Verification items for the finished model (mm, model axes). A direction names the side the tool comes from. Give positions to 0.01 mm unless a question says otherwise; leave off trailing zeros. Order: outer loops, then holes, each group sorted by start corner. A loop starts at its lowest first (then second) coordinate and runs counter-clockwise, first axis right, second up. Notation, with made-up numbers: (41.25, -13) -> (49.25, -13) arc R16 cw to (49.25, -6) -> close; hole circle Ø6 at (-32, -3.75). An arc over 180 degrees is marked (long way). Write each question's results on one line, items separated by ' | '. Start each with the question number.
1. Set-up check for faces 1 (the face through (2.5, 1, 3)), 2 (the face through (25.5, 1, 3)), 3 (the face through (22.024, 1.014, 2.283)): record each of +Z, -Z, +X, -X, +Y, -Y from which the full face is reachable in a straight line by a thin tool's end or side.
2. Cross-section at A-A, the plane x = 23. Enter the section's corners in (y, z), then the cut area to 3 significant figures.
3. Cross-section at D-D, the plane x = 5. Enter the section's corners in (y, z).
4. Material ranges on L1, parallel to X at y = 0.9, z = -3; L2, parallel to X at y = 0.85, z = -4; L3, parallel to Z at x = 5.5, y = 0.4, recorded low to high. Write a range as from..to.
5. Cross-section at B-B, the plane z = -3. Enter the section's corners in (x, y), then the cut area to 3 significant figures.
6. Depth check by flat-ended pin: pin 1 Ø0.6 at (y, z) = (1, 2) entering from -X; pin 2 Ø0.6 at (x, y) = (27, 1) entering from +Z. Enter the tip coordinate at first touch or a pass-through.
7. Cross-section at C-C, the plane y = 1.3. Enter the section's corners in (x, z), then the cut area to 3 significant figures.
8. Mould release check, pull along Z, two halves, no side actions. Record for faces 4 (the face through (0, 1, -3)), 5 (the face through (5.676, 1.014, 1.763)), 6 (the face through (15, 1, -6)), 7 (the face through (14, 1, 5)): +Z half, -Z half, draft (parallel to the pull), parting line (faces both ways), or undercut.
from build123d import *

# Parameters (mm, degrees)
SKETCH_1_W      = 30
SKETCH_1_H      = 6
SKETCH_1_R      = 1.5
EXTRUDE_1_DEPTH = 2
SKETCH_2_W      = 23
SKETCH_2_H      = 5
SKETCH_2_R      = 1
EXTRUDE_2_DEPTH = 2


with BuildPart() as part:
    # 草图1 → 凸台-拉伸1 (new body)
    with BuildSketch(Plane(origin=(0, 0, 0), x_dir=(1, 0, 0), z_dir=(0, 1, 0))):
        with Locations((15, 3)):
            Rectangle(SKETCH_1_W, SKETCH_1_H)
        with Locations(Location((5, 3, 0), (0, 0, 270))):
            Circle(SKETCH_1_R, mode=Mode.SUBTRACT)
        with Locations(Location((25, 3, 0), (0, 0, 270))):
            Circle(SKETCH_1_R, mode=Mode.SUBTRACT)
    extrude(amount=EXTRUDE_1_DEPTH)

    # 草图2 → 凸台-拉伸2 (add)
    with BuildSketch(Plane(origin=(0, 2, 0), x_dir=(1, 0, 0), z_dir=(0, 1, 0))):
        with Locations((14, -2.5)):
            Rectangle(SKETCH_2_W, SKETCH_2_H)
        with Locations(Location((5, -2.5, 0), (0, 0, 270))):
            Circle(SKETCH_2_R, mode=Mode.SUBTRACT)
        with Locations(Location((23, -2.5, 0), (0, 0, 270))):
            Circle(SKETCH_2_R, mode=Mode.SUBTRACT)
    extrude(amount=-EXTRUDE_2_DEPTH)


solid = part.part
Results below:
1) face 1: +Z, -X, +Y, -Y | face 2: +Z, +X, +Y, -Y | face 3: +Y, -Y
2) outline: (0, -6) -> (2, -6) -> (2, 1.5) -> (0, 1.5) -> close; (0, 3.5) -> (2, 3.5) -> (2, 5) -> (0, 5) -> close | area: 18.0 mm²
3) outline: (0, -6) -> (2, -6) -> (2, -4.5) -> (0, -4.5) -> close; (0, -1.5) -> (2, -1.5) -> (2, 1.5) -> (0, 1.5) -> close; (0, 3.5) -> (2, 3.5) -> (2, 5) -> (0, 5) -> close
4) L1: x = 0..3.5, 6.5..23.5, 26.5..30 | L2: x = 0..3.88, 6.12..23.88, 26.12..30 | L3: z = -6..-4.41, -1.59..1.63, 3.37..5
5) outline: (0, 0) -> (3.5, 0) -> (3.5, 2) -> (0, 2) -> close; (6.5, 0) -> (23.5, 0) -> (23.5, 2) -> (6.5, 2) -> close; (26.5, 0) -> (30, 0) -> (30, 2) -> (26.5, 2) -> close | area: 48.0 mm²
6) pin 1: stops at x = 2.5 | pin 2: stops at z = 0
7) outline: (0, -6) -> (30, -6) -> (30, 0) -> (25.5, 0) -> (25.5, 5) -> (2.5, 5) -> (2.5, 0) -> (0, 0) -> close; hole circle Ø3 at (5, -3); hole circle Ø2 at (5, 2.5); hole circle Ø2 at (23, 2.5); hole circle Ø3 at (25, -3) | area: 275 mm²
8) face 4: draft | face 5: undercut | face 6: -Z half | face 7: +Z half
